The figure shows three views and two pictorial views of one solid part (mm, origin at its lowest corner). Answer the questions. Coordinates: 2 decimals unless noted, no trailing zeros. Loops run counter-clockwise (first coordinate to the right, second up) from the corner with the lowest first, then second, coordinate; pieces in that order, holes last. Notation, with made-up numbers: M 34,69 L 78,69 A32 cw 78,108 Z; hole C 73,86.25 d10. An arc over 180 degrees is marked long. Return JSON: item names as keys, results as strings. Group by question number.
1. The mould has two halves that part along Y. Classify the marked faces 1, 2 and 3: pulls with the +Y half, pulls with the -Y half, needs draft (parallel to the pull), parting line crosses it, or undercut.
2. Section D-D (z = 8.5) is taken. Write down the section's boundary in (x, y).
3. Straight lines are drawn through the part: L1, parallel to X at y = 25, z = 4.75; L2, parallel to X at y = 28, z = 4; L3, parallel to Y at x = 26, z = 9. For each, find the intervals that lie inside material, in ascending order. Write a range as from..to.
4. Section C-C (z = 4.5) is taken. Write down the section's boundary in (x, y).
5. Section A-A (y = 25) is taken. Write down the section's boundary in (x, z) (3 decimals).
6. Section B-B (x = 25) is taken. Write down the section's boundary in (y, z) (3 decimals).
7. Given P1, Ø4, axis at x = 37, y = 37.5, coming from the -Z side; P2, Ø0.6, axis at y = 30.5, z = 3, coming from the +X side; P3, Ø1, axis at x = 25, z = 4.5, coming from the +Y side; P4, Ø3, axis at y = 38.5, z = 7, coming from the +X side, each flat-ended and moving along its own axis, determine where each tip first touches the part or whether it passes through.
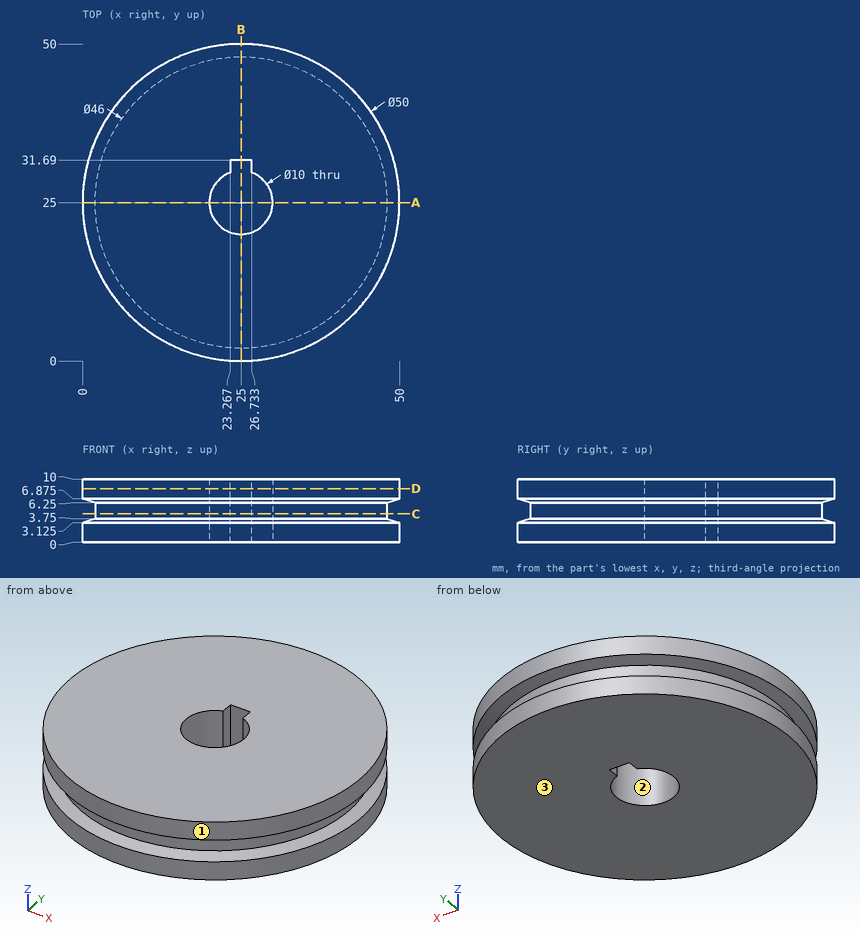
Worked out:
{
 "1": {"face 1": "parting line crosses it", "face 2": "undercut", "face 3": "needs draft"},
 "2": {"outline": "C 25,25 d50; hole M 23.27,29.69 A5 ccw long 26.73,29.69 L 26.73,31.69 L 23.27,31.69 Z"},
 "3": {"L1": "2..20, 30..48", "L2": "2.2..21, 29..47.8", "L3": "0.02..20.1, 31.69..49.98"},
 "4": {"outline": "C 25,25 d46; hole M 23.27,29.69 A5 ccw long 26.73,29.69 L 26.73,31.69 L 23.27,31.69 Z"},
 "5": {"outline": "M 0,0 L 20,0 L 20,10 L 0,10 L 0,6.875 L 2,6.25 L 2,3.75 L 0,3.125 Z; M 30,0 L 50,0 L 50,3.125 L 48,3.75 L 48,6.25 L 50,6.875 L 50,10 L 30,10 Z"},
 "6": {"outline": "M 0,0 L 20,0 L 20,10 L 0,10 L 0,6.875 L 2,6.25 L 2,3.75 L 0,3.125 Z; M 31.69,0 L 50,0 L 50,3.125 L 48,3.75 L 48,6.25 L 50,6.875 L 50,10 L 31.69,10 Z"},
 "7": {"P1": "z = 0", "P2": "x = 49.45", "P3": "y = 48", "P4": "x = 46.93"}
}
